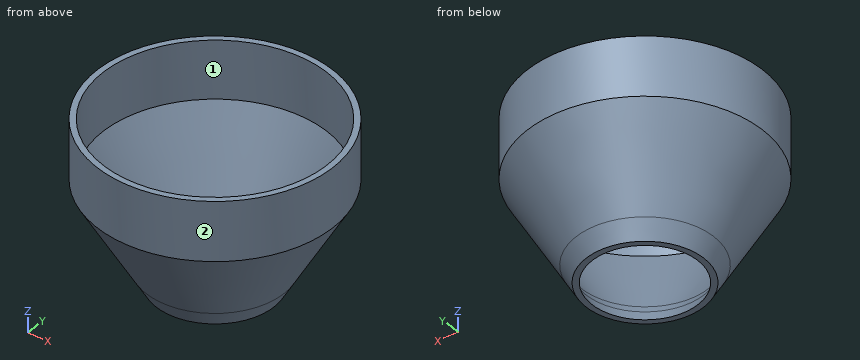
from build123d import *


with BuildPart() as f1:
    # F0 (on Front) → F1 (revolve)
    with BuildSketch(Plane.XZ):
        Polygon((-10, 0), (-9, 0), (-10, 2), align=None)
        Polygon((-11.686377, 2.906691), (-10, 0), (-10, 2), (-10.822537, 3.410457), align=None)
        Polygon((-20, 17.236307), (-11.686377, 2.906691), (-10.822537, 3.410457), (-19, 17.432883), (-19, 27.236307), (-20, 27.236307), align=None)
    revolve(axis=Axis((0, 0, 8.290515), (0, 0, 1)))


solid = f1.part
Design review of the part built by this model. Coordinates are the model's own, in mm. Face numbers are marked on the shaded views. Coordinates: 2 decimals unless noted, no trailing zeros. Order: outer loops, then holes, each group sorted by start corner. A loop starts at its lowest first (then second) coordinate and runs counter-clockwise, first axis right, second up. Notation, with made-up numbers: (-15, 29) - (43, 29) arc R36 cw to (43, 65) - close; hole circle Ø3 at (12.5, -5.75). An arc over 180 degrees is marked (long way). Put each result on its own line as item: value.
1) Wall thickness on L1, parallel to X at y = 0, z = 19.75; L2, parallel to Y at x = -13, z = 20.25: over which ranges is each line inside the solid? List them lowest first. Write a range as from..to.
Response values:
L1: x = -20..-19, 19..20
L2: y = -15.2..-13.86, 13.86..15.2
2) Take a section at B-B, the plane z = 5.25. Give the boundary of the cut face in (x, y), and give its area (3 significant figures).
Response values:
outline: circle Ø26.09 at (0, 0); hole circle Ø23.79 at (0, 0)
area: 90.2 mm²
3) The part is to be moulded in two halves that separate along Y. For the marked faces 1 and 2, say which applies: released by +Y, released by -Y, zero draft, split by the parting line, or undercut.
Response values:
face 1: undercut
face 2: split by the parting line
4) Take a section at A-A, the plane z = 24.75. Give the boundary of the cut face in (x, y).
Response values:
outline: circle Ø40 at (0, 0); hole circle Ø38 at (0, 0)
5) Insertion check: P1, Ø10, axis at x = 10.5, z = 7.5, coming from the -Y side; P2, Ø4, axis at x = 14.5, z = 14.5, coming from the -Y side; P3, Ø1, axis at y = 1.5, z = 4.5, coming from the +X side. Each pin has a flat end and moves straight along its axis. Give the tip position at first contact, or say it passes through.
Response values:
P1: stops at y = -14.89
P2: stops at y = -14.1
P3: stops at x = 12.82
